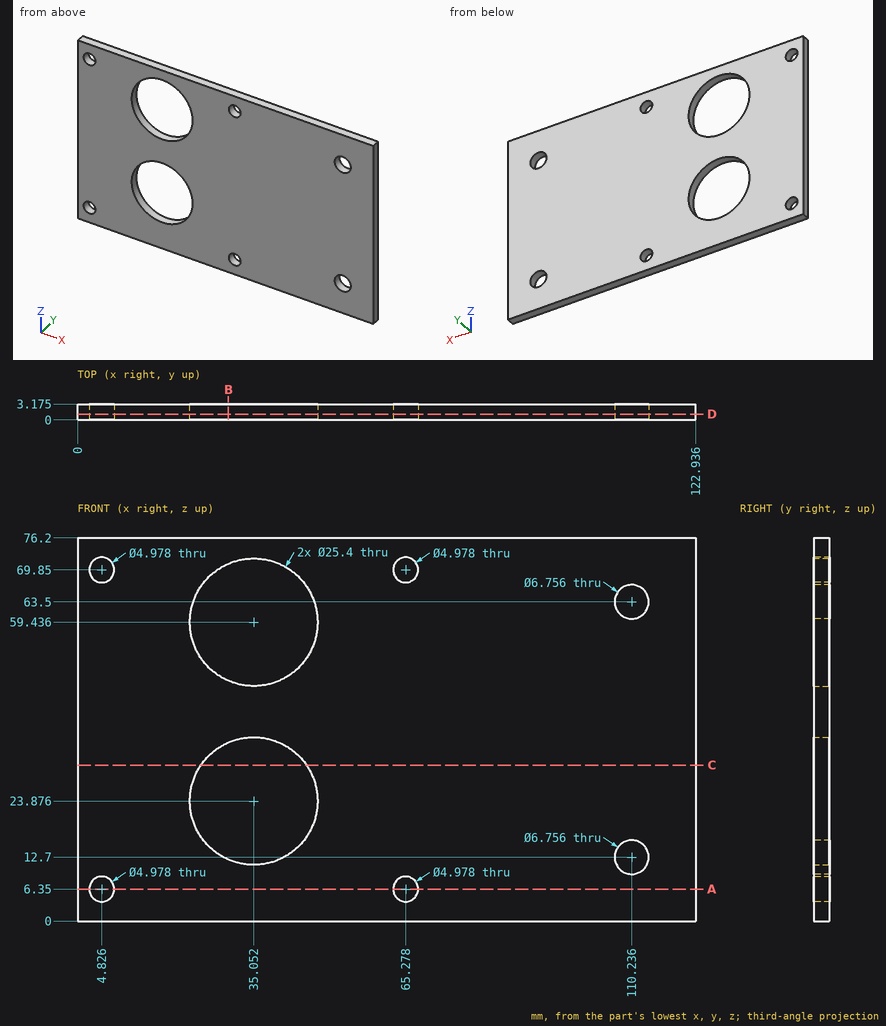
Input: dimensioned drawing with shaded views. Units: mm. Origin: part minimum x, y, z. Round coordinates to 2 decimals unless told otherwise and drop trailing zeros. Order: outer loops, then holes, each group sorted by start corner. A loop starts at its lowest first (then second) coordinate and runs counter-clockwise, first axis right, second up.
Q1. Material intervals for probe 1 along X at (y, z) = (1.7, 24.5); probe 2 along Z at (x, y) = (27, 1.65) (1 decimal); probe 3 along Z at (x, y) = (33, 2.65), sorted ascending.
Result sheet:
probe 1: x = 0 to 22.37, 47.74 to 122.94
probe 2: z = 0 to 14.1, 33.7 to 49.6, 69.3 to 76.2
probe 3: z = 0 to 11.34, 36.41 to 46.9, 71.97 to 76.2
Q2. Section B-B, the plane x = 30. Output: boundary loops of the cut face in (y, z) (1 decimal).
Result sheet:
outline: (0, 0) - (3.2, 0) - (3.2, 12.2) - (0, 12.2) - close; (0, 35.5) - (3.2, 35.5) - (3.2, 47.8) - (0, 47.8) - close; (0, 71.1) - (3.2, 71.1) - (3.2, 76.2) - (0, 76.2) - close
Q3. Section D-D, the plane y = 1.15. Give the number of separate pieces and of enclosed holes in the cut face.
Result sheet:
separate pieces: 1
enclosed holes: 8
Q4. Section A-A, the plane z = 6.35. Output: boundary loops of the cut face in (x, y) (1 decimal).
Result sheet:
outline: (0, 0) - (2.3, 0) - (2.3, 3.2) - (0, 3.2) - close; (7.3, 0) - (62.8, 0) - (62.8, 3.2) - (7.3, 3.2) - close; (67.8, 0) - (122.9, 0) - (122.9, 3.2) - (67.8, 3.2) - close
Q5. Pin query (flat end, axial travel): pin 1 (4.5 mm diameter, centred on x = 65.278, z = 6.35, fed in from -Y). Return the tip coordinate at first contact, or that it passes through.
Result sheet:
pin 1: passes through
Q6. Section C-C, the plane z = 31. Output: boundary loops of the cut face in (x, y) (1 decimal).
Result sheet:
outline: (0, 0) - (24.5, 0) - (24.5, 3.2) - (0, 3.2) - close; (45.6, 0) - (122.9, 0) - (122.9, 3.2) - (45.6, 3.2) - close
